from build123d import *

# Parameters (mm, degrees)
SKETCH1_W           = 40.2
SKETCH1_H           = 51.35
BOSS_EXTRUDE1_DEPTH = 5
BOSS_EXTRUDE2_DEPTH = 12.295
SKETCH4_R           = 1.249999996
SKETCH4_R_2         = 1.249999994
CUT_EXTRUDE1_DEPTH  = 10


with BuildPart() as part:
    # Sketch1 → Boss-Extrude1 (new body)
    with BuildSketch(Plane.XY):
        with Locations((-33.356876364, -1261.35554294)):
            Rectangle(SKETCH1_W, SKETCH1_H)
    extrude(amount=BOSS_EXTRUDE1_DEPTH)

    # Sketch2 → Boss-Extrude2 (add)
    with BuildSketch(Plane.XY.offset(5)):
        Polygon((-53.456876364, -1281.53054294), (-53.456876364, -1283.03054294), (-53.456876364, -1284.53054294), (-13.256876364, -1284.53054294), (-13.256876364, -1281.53054294), align=None)
    extrude(amount=BOSS_EXTRUDE2_DEPTH)

    # Sketch4 → Cut-Extrude1 (cut)
    with BuildSketch(Plane.XY.offset(5)):
        with Locations((-45.256876364, -1276.030542925)):
            Circle(SKETCH4_R)
        with Locations((-37.256876364, -1276.030542925)):
            Circle(SKETCH4_R_2)
        with Locations((-29.256876364, -1276.03054293)):
            Circle(SKETCH4_R)
        with Locations((-21.26485567, -1276.03054293)):
            Circle(SKETCH4_R)
    extrude(amount=-CUT_EXTRUDE1_DEPTH, mode=Mode.SUBTRACT)


solid = part.part
Geometry check sheet. Reference: the model listing, model coordinates, mm. A direction names the side the tool comes from. Give positions to 0.01 mm unless a question says otherwise; leave off trailing zeros. Order: outer loops, then holes, each group sorted by start corner. A loop starts at its lowest first (then second) coordinate and runs counter-clockwise, first axis right, second up.
1) Draft check along X on faces 1 (the cylindrical face through (-44.58, -1274.98, 2.54)), 2 (the flat face through (-34, -1261, 0)), 3 (the flat face through (-13.257, -1265, 4)). Enter one of: released by +X, released by -X, zero draft, split by the parting line, or undercut.
Results are:
face 1: undercut
face 2: zero draft
face 3: released by +X
2) Cross-section at D-D (z = 9.5). Record the boundary of the cut face in (x, y), then the cut area to 3 significant figures.
Results are:
outline: (-53.46, -1284.53) - (-13.26, -1284.53) - (-13.26, -1281.53) - (-53.46, -1281.53) - close
area: 121 mm2
3) Cross-section at A-A (x = -49). Record the boundary of the cut face in (y, z) (3 decimals), then the cut area to 3 significant figures.
Results are:
outline: (-1287.031, 0) - (-1235.681, 0) - (-1235.681, 5) - (-1281.531, 5) - (-1281.531, 17.295) - (-1284.531, 17.295) - (-1284.531, 5) - (-1287.031, 5) - close
area: 294 mm2
4) Cross-section at B-B (x = -29). Record the boundary of the cut face in (y, z) (3 decimals), then the cut area to 3 significant figures.
Results are:
outline: (-1287.031, 0) - (-1277.254, 0) - (-1277.254, 5) - (-1281.531, 5) - (-1281.531, 17.295) - (-1284.531, 17.295) - (-1284.531, 5) - (-1287.031, 5) - close; (-1274.807, 0) - (-1235.681, 0) - (-1235.681, 5) - (-1274.807, 5) - close
area: 281 mm2
5) Material ranges on probe 1 along Z at (x, y) = (-18.5, -1271); probe 2 along X at (y, z) = (-1276.5, 1.5); probe 3 along Y at (x, z) = (-41, 13), recorded low to high.
Results are:
probe 1: z = 0 to 5
probe 2: x = -53.46 to -46.42, -44.1 to -38.42, -36.1 to -30.42, -28.1 to -22.42, -20.11 to -13.26
probe 3: y = -1284.53 to -1281.53
6) Cross-section at C-C (y = -1250). Record the boundary of the cut face in (x, z).
Results are:
outline: (-53.46, 0) - (-13.26, 0) - (-13.26, 5) - (-53.46, 5) - close
7) Tool access check on faces 4 (the flat face through (-34, -1287.031, 2)), 5 (the flat face through (-34, -1284.531, 11)), 6 (the flat face through (-34, -1258, 5)). Record the directions out of +Z, -Z, +X, -X, +Y, -Y that give a thin tool (end or side, any length) a straight path to the whole face; none if there is none.
Results are:
face 4: +Z, -Z, +X, -X, -Y
face 5: +Z, +X, -X, -Y
face 6: +Z, +X, -X, +Y
8) Gauge pin test, flat ends, axial feed: pin 1 (3 mm diameter, centred on x = -35.5, z = 9, fed in from +Y); pin 2 (2 mm diameter, centred on x = -45.26, y = -1276.03, fed in from +Z); pin 3 (5 mm diameter, centred on x = -30.5, y = -1271.5, fed in from +Z); pin 4 (3.5 mm diameter, centred on x = -40.5, z = 10.5, fed in from -Y). Record the tip position at first contact, or that the pin passes through.
Results are:
pin 1: stops at y = -1281.53
pin 2: passes through
pin 3: stops at z = 5
pin 4: stops at y = -1284.53
